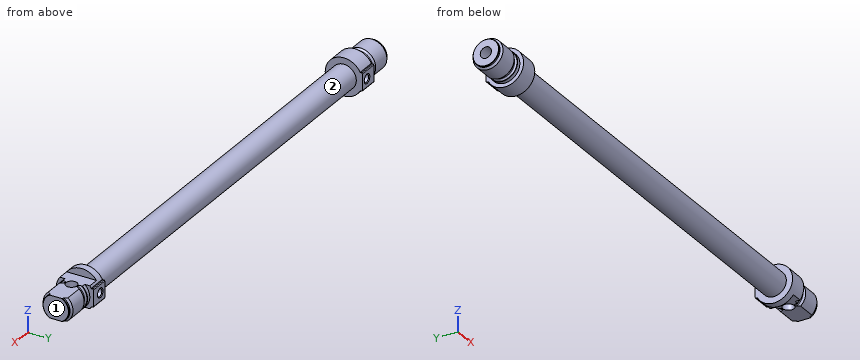
Autodesk Inventor part; units mm, degrees
ref_plane "FDT_FRONT_XY" through (17, 0, 0) normal (1, 0, 0) x (0, 0, -1)
ref_plane "FDT_FRONT_YZ" through (17, 0, 0) normal (0, 0, -1) x (0, 1, 0)
ref_plane "FDT_FRONT_ZX" through (17, 0, 0) normal (0, 1, 0) x (1, 0, 0)
sketch "Sketch_1" plane through (0, 0, 0) normal (0, 0, 1) x (1, 0, 0)
  line L0 (17, 0) -> (0, 0)
  line L1 (0, 0) -> (0, 6.8)
  line L2 (0, 6.8) -> (0.2, 7)
  line L3 (0.2, 7) -> (1, 7)
  line L4 (1, 7) -> (2, 8)
  line L5 (2, 8) -> (11.95, 8)
  line L6 (11.95, 8) -> (12.8657, 7.0843)
  arc A0 (12.8657, 7.0843) -> (13.4314, 6.85) centre (13.4314, 7.65) ccw
  line L7 (13.4314, 6.85) -> (14.2, 6.85)
  arc A1 (14.2, 6.85) -> (15, 7.65) centre (14.2, 7.65) ccw
  line L8 (15, 7.65) -> (15, 8)
  line L9 (15, 8) -> (17, 8)
  line L10 (17, 8) -> (17, 0)
  line L11 (17, 0) -> (0, 0)
revolve "Revolution1" add sketch "Sketch_1" angle 360 about axis through (17, 0, 0) along (1, 0, 0)
thread "Thread1"
sketch "Sketch_2" plane through (17, 0, 0) normal (1, 0, 0) x (0, 0, -1)
  arc A0 (-4.9029, 8.7156) -> (4.9029, 8.7156) centre (0, 0) ccw
  arc A1 (4.75, 8.9771) -> (4.9029, 8.7156) centre (5.05, 8.9771) ccw
  line L0 (4.75, 8.9771) -> (4.75, 9.6)
  arc A2 (4.75, 9.6) -> (4.35, 10) centre (4.35, 9.6) ccw
  line L1 (4.35, 10) -> (-4.35, 10)
  arc A3 (-4.35, 10) -> (-4.75, 9.6) centre (-4.35, 9.6) ccw
  line L2 (-4.75, 9.6) -> (-4.75, 8.9771)
  arc A4 (-4.9029, 8.7156) -> (-4.75, 8.9771) centre (-5.05, 8.9771) ccw
extrude "Extrusion1" add sketch "Sketch_2" along normal blind 10
sketch "Sketch_3" plane through (0, 0, 0) normal (0, 0, 1) x (1, 0, 0)
  line L0 (257, 0) -> (27, 0)
  line L1 (27, 0) -> (27, 6.65)
  line L2 (27, 6.65) -> (257, 6.65)
  line L3 (257, 6.65) -> (257, 0)
  line L4 (257, 0) -> (27, 0)
revolve "Revolution2" add sketch "Sketch_3" angle 360 about axis through (257, 0, 0) along (1, 0, 0)
sketch "Sketch_16" plane through (257, 0, 0) normal (1, 0, 0) x (0, 0, -1)
  arc A0 (-4.9029, 8.7156) -> (4.9029, 8.7156) centre (0, 0) ccw
  arc A1 (4.75, 8.9771) -> (4.9029, 8.7156) centre (5.05, 8.9771) ccw
  line L0 (4.75, 8.9771) -> (4.75, 9.6)
  arc A2 (4.75, 9.6) -> (4.35, 10) centre (4.35, 9.6) ccw
  line L1 (4.35, 10) -> (-4.35, 10)
  arc A3 (-4.35, 10) -> (-4.75, 9.6) centre (-4.35, 9.6) ccw
  line L2 (-4.75, 9.6) -> (-4.75, 8.9771)
  arc A4 (-4.9029, 8.7156) -> (-4.75, 8.9771) centre (-5.05, 8.9771) ccw
extrude "Extrusion2" add sketch "Sketch_16" along normal blind 10
sketch "Sketch_23" plane through (0, 0, 0) normal (0, 0, 1) x (1, 0, 0)
  line L0 (284, 0) -> (267, 0)
  line L1 (267, 0) -> (267, 8)
  line L2 (267, 8) -> (269, 8)
  line L3 (269, 8) -> (269, 7.65)
  arc A0 (269, 7.65) -> (269.8, 6.85) centre (269.8, 7.65) ccw
  line L4 (269.8, 6.85) -> (270.5686, 6.85)
  arc A1 (270.5686, 6.85) -> (271.1343, 7.0843) centre (270.5686, 7.65) ccw
  line L5 (271.1343, 7.0843) -> (272.05, 8)
  line L6 (272.05, 8) -> (282, 8)
  line L7 (282, 8) -> (283, 7)
  line L8 (283, 7) -> (283.8, 7)
  line L9 (283.8, 7) -> (284, 6.8)
  line L10 (284, 6.8) -> (284, 0)
  line L11 (284, 0) -> (267, 0)
revolve "Revolution3" add sketch "Sketch_23" angle 360 about axis through (284, 0, 0) along (1, 0, 0)
thread "Thread2"
sketch "Sketch_6" plane through (0, 0, 0) normal (0, 1, 0) x (-1, 0, 0)
  line L0 (-261, -18) -> (-261, -6)
  line L1 (-261, -6) -> (-284, -6)
  line L2 (-284, -6) -> (-284, 6)
  line L3 (-284, 6) -> (-261, 6)
  line L4 (-261, 6) -> (-261, 18)
  line L5 (-261, 18) -> (-296, 18)
  line L6 (-296, 18) -> (-296, -18)
  line L7 (-296, -18) -> (-261, -18)
extrude "Extrusion3" cut sketch "Sketch_6" along normal mid plane 20
sketch "Sketch7" plane through (282, -5.2915, -6) normal (0, 0, -1) x (-1, 0, 0)
  point P0 (12, 5.2915)
hole "Hole1" at (270, 0, -6) direction (0, 0, 1) diameter 6 depth 12
sketch "Sketch8" plane through (17, 10, 4.35) normal (0, 1, 0) x (1, 0, 0)
  point P0 (6, 4.35)
hole "Hole2" at (23, 10, 0) direction (0, -1, 0) diameter 4.134 depth 10 countersink diameter 5 countersink angle 90
sketch "Sketch9" plane through (257, 10, 4.35) normal (0, 1, 0) x (1, 0, 0)
  point P0 (4, 4.35)
hole "Hole3" at (261, 10, 0) direction (0, -1, 0) diameter 4.134 depth 11 tip angle 120 countersink diameter 5 countersink angle 90
sketch "Sketch_64" plane through (0, 0, 0) normal (0, 0, 1) x (1, 0, 0)
  line L0 (240.3, 0) -> (-5, 0)
  line L1 (-5, 0) -> (-5, 3)
  line L2 (-5, 3) -> (37.3, 3)
  line L3 (37.3, 3) -> (37.3, 6)
  line L4 (37.3, 6) -> (240.3, 6)
  line L5 (240.3, 6) -> (240.3, 0)
  line L6 (240.3, 0) -> (-5, 0)
revolve "Revolution4" cut sketch "Sketch_64" angle 360 about axis through (240.3, 0, 0) along (1, 0, 0)
ref_plane "FDT_FRONT_XY" through (17, 0, 0) normal (1, 0, 0) x (0, 0, -1)
ref_plane "FDT_FRONT_YZ" through (17, 0, 0) normal (0, 0, -1) x (0, 1, 0)
ref_plane "FDT_FRONT_ZX" through (17, 0, 0) normal (0, 1, 0) x (1, 0, 0)
ref_plane "FDT_QSFRONT_XY" through (23, 10, 0) normal (0, 1, 0) x (0, 0, 1)
ref_plane "FDT_QSFRONT_YZ" through (23, 10, 0) normal (0, 0, 1) x (1, 0, 0)
ref_plane "FDT_QSFRONT_ZX" through (23, 10, 0) normal (1, 0, 0) x (0, 1, 0)
ref_plane "FDT_QSREAR_XY" through (261, 10, 0) normal (0, 1, 0) x (0, 0, 1)
ref_plane "FDT_QSREAR_YZ" through (261, 10, 0) normal (0, 0, 1) x (1, 0, 0)
ref_plane "FDT_QSREAR_ZX" through (261, 10, 0) normal (1, 0, 0) x (0, 1, 0)
ref_plane "FDT_REAR_XY" through (267, 0, 0) normal (-1, 0, 0) x (0, 0, -1)
ref_plane "FDT_REAR_YZ" through (267, 0, 0) normal (0, 0, -1) x (0, -1, 0)
ref_plane "FDT_REAR_ZX" through (267, 0, 0) normal (0, -1, 0) x (-1, 0, 0)
ref_plane "FDT_SMBR1_XY" through (36.5, 0, 0) normal (-1, 0, 0) x (0, 0, 1)
ref_plane "FDT_SMBR1_YZ" through (36.5, 0, 0) normal (0, 0, 1) x (0, 1, 0)
ref_plane "FDT_SMBR1_ZX" through (36.5, 0, 0) normal (0, 1, 0) x (-1, 0, 0)
ref_plane "FDT_SMBR2_XY" through (247.5, 0, 0) normal (-1, 0, 0) x (0, 0, 1)
ref_plane "FDT_SMBR2_YZ" through (247.5, 0, 0) normal (0, 0, 1) x (0, 1, 0)
ref_plane "FDT_SMBR2_ZX" through (247.5, 0, 0) normal (0, 1, 0) x (-1, 0, 0)
ref_plane "FDT_SWIVELAXIS_XY" through (270, 0, 0) normal (0, 0, 1) x (1, 0, 0)
ref_plane "FDT_SWIVELAXIS_YZ" through (270, 0, 0) normal (1, 0, 0) x (0, 1, 0)
ref_plane "FDT_SWIVELAXIS_ZX" through (270, 0, 0) normal (0, 1, 0) x (0, 0, 1)
ref_plane "NUT_XY" through (8, 0, 0) normal (1, 0, 0) x (0, 0, -1)
ref_plane "NUT_YZ" through (8, 0, 0) normal (0, 0, -1) x (0, 1, 0)
ref_plane "NUT_ZX" through (8, 0, 0) normal (0, 1, 0) x (1, 0, 0)
ref_plane "ZR_XY" through (0, 0, 0) normal (1, 0, 0) x (0, 0, -1)
ref_plane "ZR_YZ" through (0, 0, 0) normal (0, 0, -1) x (0, 1, 0)
ref_plane "ZR_ZX" through (0, 0, 0) normal (0, 1, 0) x (1, 0, 0)
ref_plane "ZYL_XY" through (17, 0, 0) normal (1, 0, 0) x (0, 0, -1)
ref_plane "ZYL_YZ" through (17, 0, 0) normal (0, 0, -1) x (0, 1, 0)
ref_plane "ZYL_ZX" through (17, 0, 0) normal (0, 1, 0) x (1, 0, 0)
properties part number "19197 DSNU-12-200-P---(A----0-ZR)"
Part model, mm, in its own coordinate system. Face numbers are marked on the shaded views. Coordinates: 2 decimals unless noted, no trailing zeros. Write each loop counter-clockwise with the first axis right and the second up, starting at its lowest first coordinate (ties: lowest second). Pieces come first, ordered by that corner, then holes. Notation, with made-up numbers: M -26.75,71 L -2.75,71 A16 cw -2.75,81 Z; hole C -15,87.5 d7. An arc over 180 degrees is marked long. Return JSON: item names as keys, results as strings.
1. Probe L1, parallel to X at y = -0.5, z = 5; L2, parallel to Z at x = 25.5, y = 0; L3, parallel to Z at x = 23, y = 6.5. List the from-to ranges inside material, lowest first.
Determined:
{"L1": "0 to 37.3, 240.3 to 267.04, 272.96 to 284", "L2": "-10 to -3, 3 to 10", "L3": "-7.6 to -2.07, 2.07 to 7.6"}
2. Saw through at A-A, the plane x = 94. Write the cut outline in (y, z).
Determined:
{"outline": "C 0,0 d13.3; hole C 0,0 d12"}
3. Pull direction X, two halves, no side cores. Call the marked faces 1 and 2: pulls with the +X half, pulls with the -X half, needs draft (parallel to the pull), parting line crosses it, or undercut.
Determined:
{"face 1": "pulls with the +X half", "face 2": "undercut"}
4. Flat gauge pins, fed straight in: pin 1 Ø8 at (x, y) = (71, 0.5) entering from -Z; pin 2 Ø6 at (x, z) = (177, 0.5) entering from -Y; pin 3 Ø2 at (x, z) = (91, 5) entering from +Y. Where does each tip first touch, or does it go through?
Determined:
{"pin 1": "z = -6.65", "pin 2": "y = -6.65", "pin 3": "y = 5.31"}
